```python
from build123d import *

# Parameters (mm, degrees)
F0_R     = 2
F0_W     = 51
F0_H     = 73.2
F1_DEPTH = 13.5
F2_R     = 5
F3_SIZE  = 2


with BuildPart() as f1:
    # F0 (on Top) → F1 (new body)
    with BuildSketch(Plane.XY):
        Polygon((28.5, -5), (28.5, 5), (-28.5, 5), (-28.5, -5), (-28.5, -78.2), (-28.5, -88.2), (28.5, -88.2), (28.5, -78.2), align=None)
        with Locations((0, -83.2)):
            Circle(F0_R, mode=Mode.SUBTRACT)
        with Locations((0, -41.6)):
            Rectangle(F0_W, F0_H, mode=Mode.SUBTRACT)
        Circle(F0_R, mode=Mode.SUBTRACT)
    extrude(amount=F1_DEPTH)

    # F2
    f2_edges = [f1.edges().sort_by_distance(p)[0] for p in [
        (-28.5, 5, 6.75),
        (28.5, 5, 6.75),
        (-28.5, -88.2, 6.75),
        (28.5, -88.2, 6.75),
    ]]
    fillet(f2_edges, radius=F2_R)

    # F3
    f3_edges = [f1.edges().sort_by_distance(p)[0] for p in [
        (-2, 0, 13.5),
        (-2, -83.2, 13.5),
    ]]
    chamfer(f3_edges, length=F3_SIZE)


solid = f1.part
```
Verification items for the finished model (mm, model axes). A direction names the side the tool comes from. Give positions to 0.01 mm unless a question says otherwise; leave off trailing zeros. Loops run counter-clockwise (first coordinate to the right, second up) from the corner with the lowest first, then second, coordinate; pieces in that order, holes last. Notation, with made-up numbers: M 83,-30.75 L 138,-30.75 A19 cw 138,-2.75 Z; hole C 61,87.25 d4. An arc over 180 degrees is marked long. Return JSON: item names as keys, results as strings.
1) Section check D-D, the plane z = 7.5. Enter the section's corners in (x, y), and give its area (3 significant figures).
Findings:
{"outline": "M -28.5,-83.2 A5 ccw -23.5,-88.2 L 23.5,-88.2 A5 ccw 28.5,-83.2 L 28.5,0 A5 ccw 23.5,5 L -23.5,5 A5 ccw -28.5,0 Z; hole M -25.5,-78.2 L 25.5,-78.2 L 25.5,-5 L -25.5,-5 Z; hole C 0,-83.2 d4; hole C 0,0 d4", "area": "1,530 mm2"}
2) Tool access check on faces 4 (the flat face through (-25.5, -42, 7)), 5 (the cylindrical face through (-27.07, -86.7, 6.84)). Record the directions out of +Z, -Z, +X, -X, +Y, -Y that give a thin tool (end or side, any length) a straight path to the whole face; none if there is none.
Findings:
{"face 4": "+Z, -Z", "face 5": "+Z, -Z, -X, -Y"}
3) Mould release check, pull along X, two halves, no side actions. Record for faces 1 (the flat face through (0, -5, 7)), 2 (the cylindrical face through (27.07, -86.7, 6.84)), 3 (the flat face through (27, -41, 0)): released by +X, released by -X, zero draft, split by the parting line, or undercut.
Findings:
{"face 1": "undercut", "face 2": "released by +X", "face 3": "zero draft"}
4) Gauge pin test, flat ends, axial feed: P1, Ø5, axis at x = 0, y = 0, coming from the +Z side; P2, Ø6.5, axis at x = 0, y = -83.2, coming from the +Z side; P3, Ø10, axis at x = -16.5, y = -28.5, coming from the -Z side. Record the tip position at first contact, or that the pin passes through.
Findings:
{"P1": "stops at z = 12", "P2": "stops at z = 12.75", "P3": "passes through"}
5) Section check B-B, the plane y = -66. Enter the section's corners in (x, z), and give its area (3 significant figures).
Findings:
{"outline": "M -28.5,0 L -25.5,0 L -25.5,13.5 L -28.5,13.5 Z; M 25.5,0 L 28.5,0 L 28.5,13.5 L 25.5,13.5 Z", "area": "81.0 mm2"}
6) Section check A-A, the plane x = 0. Enter the section's corners in (y, z), and give its area (3 significant figures).
Findings:
{"outline": "M -88.2,0 L -85.2,0 L -85.2,11.5 L -87.2,13.5 L -88.2,13.5 Z; M -81.2,0 L -78.2,0 L -78.2,13.5 L -79.2,13.5 L -81.2,11.5 Z; M -5,0 L -2,0 L -2,11.5 L -4,13.5 L -5,13.5 Z; M 2,0 L 5,0 L 5,13.5 L 4,13.5 L 2,11.5 Z", "area": "154 mm2"}
7) Section check C-C, the plane x = -15. Enter the section's corners in (y, z), and give its area (3 significant figures).
Findings:
{"outline": "M -88.2,0 L -78.2,0 L -78.2,13.5 L -88.2,13.5 Z; M -5,0 L 5,0 L 5,13.5 L -5,13.5 Z", "area": "270 mm2"}
8) Material ranges on L1, parallel to Y at x = 0, z = 6; L2, parallel to Y at x = -11.5, z = 4.5; L3, parallel to X at y = -52, z = 12, recorded low to high. Write a range as [from, to].
Findings:
{"L1": "y = [-88.2, -85.2], [-81.2, -78.2], [-5, -2], [2, 5]", "L2": "y = [-88.2, -78.2], [-5, 5]", "L3": "x = [-28.5, -25.5], [25.5, 28.5]"}
